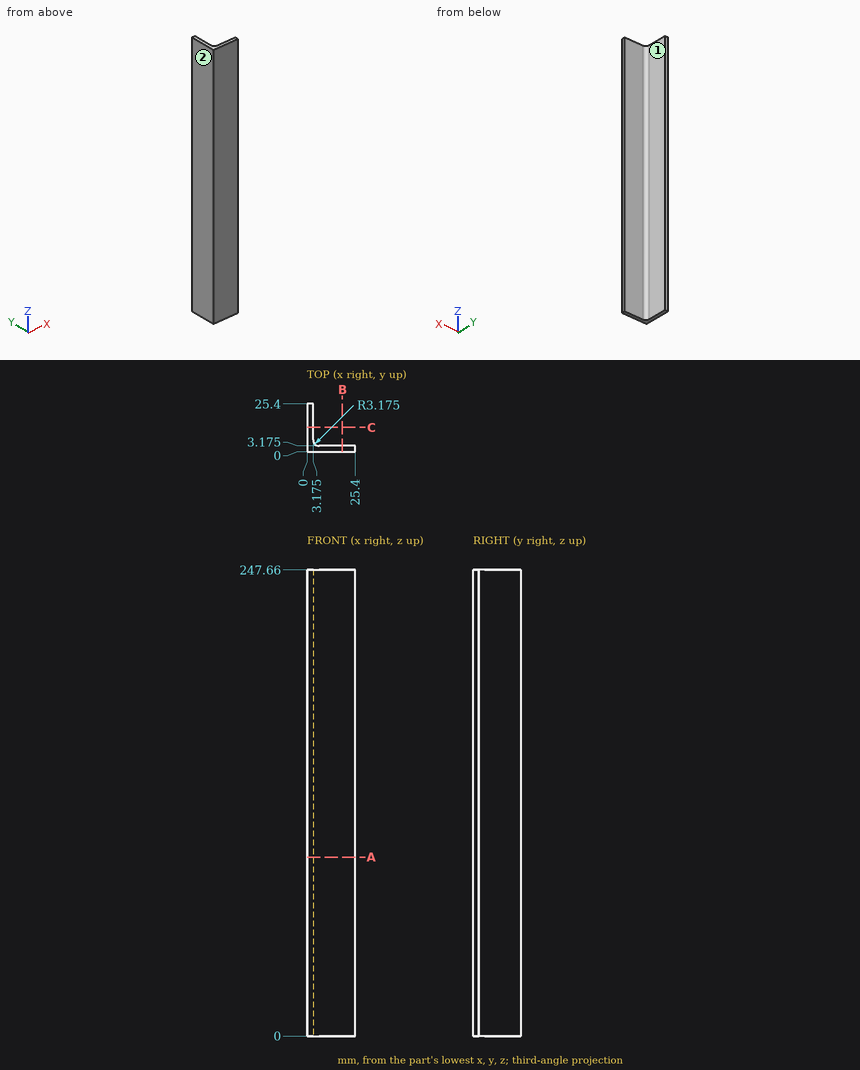
Geometry: see drawing. Coordinates: mm, zero at the bounding-box minimum. A direction names the side the tool comes from. Give positions to 0.01 mm unless a question says otherwise; leave off trailing zeros. Write each loop counter-clockwise with the first axis right and the second up, starting at its lowest first coordinate (ties: lowest second). Pieces come first, ordered by that corner, then holes. Notation, with made-up numbers: M 3.25,5.5 L 17.25,5.5 A10 cw 17.25,15.5 Z; hole C 57.5,55.25 d2. An arc over 180 degrees is marked long. Return JSON: item names as keys, results as strings. Group by question number.
1) Cut plane A-A, the plane z = 95. Output: boundary loops of the cut face in (x, y) (3 decimals).
2) Cut plane B-B, the plane x = 18.75. Output: boundary loops of the cut face in (y, z) (3 decimals).
3) First-contact query: pin 1 Ø6 at (x, y) = (4.5, 14.5) entering from -Z; pin 2 Ø9.5 at (y, z) = (18.5, 155) entering from +X (3 decimals); pin 3 Ø15 at (x, z) = (14.5, 67.5) entering from +Y (3 decimals). Flat tips, straight axial feed; report the tip coordinate or a pass-through.
4) Set-up query: the marked faces 1 and 2. Return all of +Z, -Z, +X, -X, +Y, -Y with unobstructed straight access to the full face (end or side cutting, diameter ignored); none if empty.
5) Ray query, L1, parallel to Y at x = 23, z = 58.5 (3 decimals); L2, parallel to Y at x = 4.5, z = 14. Return the intervals inside material, ascending.
Data:
{
 "1": {"outline": "M 0,0 L 25.4,0 L 25.4,3.175 L 6.35,3.175 A3.175 cw 3.175,6.35 L 3.175,25.4 L 0,25.4 Z"},
 "2": {"outline": "M 0,0 L 3.175,0 L 3.175,247.66 L 0,247.66 Z"},
 "3": {"pin 1": "stops at z = 0", "pin 2": "stops at x = 3.175", "pin 3": "stops at y = 3.175"},
 "4": {"face 1": "+Z, -Z, +X, +Y", "face 2": "+Z, -Z, -X, +Y, -Y"},
 "5": {"L1": "y = 0 to 3.175", "L2": "y = 0 to 3.77"}
}
